For this review, take the finished solid that the model builds, in its own axes (mm). Coordinates: 2 decimals unless noted, no trailing zeros. Write each loop counter-clockwise with the first axis right and the second up, starting at its lowest first coordinate (ties: lowest second). Pieces come first, ordered by that corner, then holes. Notation, with made-up numbers: (-30, -4.5) -> (13, -4.5) arc R34 ccw to (13, 34.5) -> close; hole circle Ø4 at (68.5, 7.5). An arc over 180 degrees is marked (long way). One line per item, written item: value. Start each with the question number.
1) For probe 1 along Z at (x, y) = (120.65, 0.75); probe 2 along X at (y, z) = (-1.75, 1.25), list the stretches that pass through material, from the lowest coordinate up. Write a range as from..to.
2) Add section A-A (y = -1.5). State the section outline as (x, z) points.
3) For pin 1 Ø1.5 at (y, z) = (0, 4.5) entering from -X, flat-tipped, find the tip position at first contact; note if it passes through.
4) Add section B-B (z = 2). State the section outline as (x, y) points (3 decimals), and give its area (3 significant figures).
from build123d import *

# Parameters (mm, degrees)
F0_R     = 3.96875
F1_DEPTH = 3.175


with BuildPart() as f1:
    # F0 (on Front) → F1 (new body, symmetric)
    with BuildSketch(Plane.XZ):
        with BuildLine():
            Line((120.65, 6.35), (-120.65, 6.35))
            ThreePointArc((-120.65, 6.35), (-125.140128, 4.490128), (-127, 0))
            ThreePointArc((-127, 0), (-125.140128, -4.490128), (-120.65, -6.35))
            Line((-120.65, -6.35), (120.65, -6.35))
            ThreePointArc((120.65, -6.35), (125.140128, -4.490128), (127, 0))
            ThreePointArc((127, 0), (125.140128, 4.490128), (120.65, 6.35))
        make_face()
        with Locations((-120.65, 0)):
            Circle(F0_R, mode=Mode.SUBTRACT)
        with Locations((120.65, 0)):
            Circle(F0_R, mode=Mode.SUBTRACT)
    extrude(amount=F1_DEPTH, both=True)


solid = f1.part
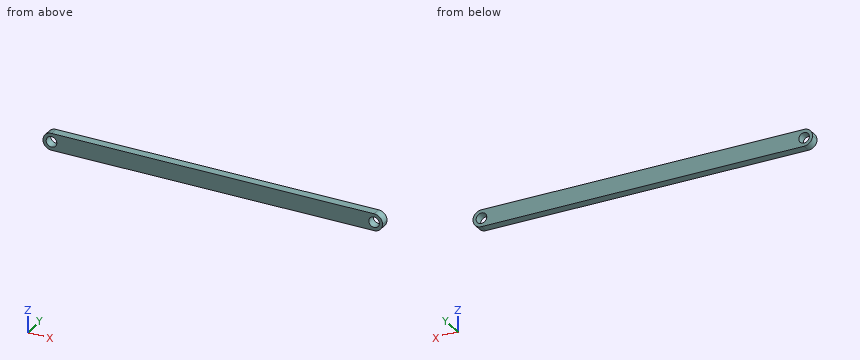
Numbers:
1. probe 1: -6.35..-3.97, 3.97..6.35
1. probe 2: -126.88..-124.42, -116.88..116.88, 124.42..126.88
2. outline: (-120.65, -6.35) -> (120.65, -6.35) arc R6.35 ccw to (120.65, 6.35) -> (-120.65, 6.35) arc R6.35 ccw to start; hole circle Ø7.94 at (-120.65, 0); hole circle Ø7.94 at (120.65, 0)
3. pin 1: x = -125.77
4. outline: (-126.677, -3.175) -> (-124.078, -3.175) -> (-124.078, 3.175) -> (-126.677, 3.175) -> close; (-117.222, -3.175) -> (117.222, -3.175) -> (117.222, 3.175) -> (-117.222, 3.175) -> close; (124.078, -3.175) -> (126.677, -3.175) -> (126.677, 3.175) -> (124.078, 3.175) -> close
4. area: 1,520 mm²
